Geometry: final body of the model. Coordinates: model frame, mm. A direction names the side the tool comes from. Give positions to 0.01 mm unless a question says otherwise; leave off trailing zeros. Write each loop counter-clockwise with the first axis right and the second up, starting at its lowest first coordinate (ties: lowest second). Pieces come first, ordered by that corner, then holes. Notation, with made-up numbers: M 86.5,66 L 106.5,66 A12 cw 106.5,85 Z; hole C 53,-28.5 d9. An arc over 180 degrees is marked long. Answer as a JSON object with one key per item and string values.
from build123d import *

# Parameters (mm, degrees)
F1_DEPTH  = 16
F3_DEPTH  = 8
F5_DEPTH  = 3
F7_R      = 4.4
F6_R      = 4.55
F9_ANGLE  = 90
F10_SIZE2 = 7
F10_SIZE  = 5


with BuildPart() as f1:
    # F0 (on Top) → F1 (new body)
    with BuildSketch(Plane.XY):
        with BuildLine():
            ThreePointArc((10.125, 0), (0, 10.125), (-10.125, 0))
            Line((-10.125, 0), (-10.125, -10.125))
            Line((-10.125, -10.125), (10.125, -10.125))
            Line((10.125, -10.125), (10.125, 0))
        make_face()
    extrude(amount=F1_DEPTH)

    # F2 (on face) → F3 (cut)
    with BuildSketch(Plane.XY.offset(16)):
        with BuildLine():
            ThreePointArc((7.8, 0), (0, 7.8), (-7.8, 0))
            Line((-7.8, 0), (-7.8, -10.125))
            Line((-7.8, -10.125), (7.8, -10.125))
            Line((7.8, -10.125), (7.8, 0))
        make_face()
    extrude(amount=-F3_DEPTH, mode=Mode.SUBTRACT)

    # F4 (on face) → F5 (cut)
    with BuildSketch(Plane.XY.offset(8)):
        with BuildLine():
            ThreePointArc((9.125, 0), (0, 9.125), (-9.125, 0))
            Line((-9.125, 0), (-9.125, -10.125))
            Line((-9.125, -10.125), (9.125, -10.125))
            Line((9.125, -10.125), (9.125, 0))
        make_face()
    extrude(amount=F5_DEPTH, mode=Mode.SUBTRACT)

    # F7 (on face) → F8 section 0
    with BuildSketch(Plane(origin=(0, 0, 0), x_dir=(1, 0, 0), z_dir=(0, 0, -1))):
        Circle(F7_R)
    # F6 (on face) → F8 section 1
    with BuildSketch(Plane.XY.offset(8)):
        Circle(F6_R)
    loft(mode=Mode.SUBTRACT)


with BuildPart() as f1_1:
    # F9: moved
    add(f1.part.rotate(Axis((0, -10.125, 0), (1, 0, 0)), F9_ANGLE))

    # F10
    f10_edges = [f1_1.edges().sort_by_distance(p)[0] for p in [
        (10.125, -10.125, 5.0625),
        (0, -10.125, 20.25),
        (0, -10.125, 0),
    ]]
    f10_side = f1_1.faces().sort_by_distance((0, -10.125, 19.963622))[0]
    chamfer(f10_edges, length=F10_SIZE, length2=F10_SIZE2, reference=f10_side)


solid = f1_1.part
1) Pull-direction query (Y, two-part tool) for faces 1 (the flat face through (7.66, -13.674, 6.117)), 2 (the conical face through (-0.583, -14.181, 5.687)), 3 (the flat face through (-4, -21.125, 17)); classes: pulls with the +Y half, pulls with the -Y half, needs draft (parallel to the pull), parting line crosses it, or undercut.
Geometry check:
{"face 1": "pulls with the +Y half", "face 2": "pulls with the -Y half", "face 3": "undercut"}
2) Cut plane A-A on y = -21.75. Return loops of the section in (x, z) (3 decimals).
Geometry check:
{"outline": "M -10.125,0 L -7.8,0 L -7.8,10.125 A7.8 cw 7.8,10.125 L 7.8,0 L 10.125,0 L 10.125,10.125 A10.125 ccw -10.125,10.125 Z"}
3) Cut plane B-B on z = 4.25. Return loops of the section in (x, y) (3 decimals).
Geometry check:
{"outline": "M -10.125,-26.125 L -7.8,-26.125 L -7.8,-21.125 L -9.125,-21.125 L -9.125,-18.125 L 9.125,-18.125 L 9.125,-21.125 L 7.8,-21.125 L 7.8,-26.125 L 10.125,-26.125 L 10.125,-17.125 L 5.875,-11.175 L -5.875,-11.175 L -10.125,-17.125 Z"}
4) Set-up query: faces 4 (the cylindrical face through (0.201, -19.604, 19.248)), 5 (the flat face through (-0.8, -17.9, 0)), 6 (the flat face through (7.8, -24, 5)). Return all of +Z, -Z, +X, -X, +Y, -Y with unobstructed straight access to the full face (end or side cutting, diameter ignored); none if empty.
Geometry check:
{"face 4": "-Z", "face 5": "-Z, +X, -X, +Y, -Y", "face 6": "-Z, -Y"}
5) Contact query for flat-ended pins moving along their axis: P1, Ø2, axis at x = 1.5, z = 17.5, coming from the -Y side (3 decimals); P2, Ø4, axis at x = 3.5, y = -13.5, coming from the -Z side; P3, Ø8, axis at y = -13, z = 7, coming from the +X side; P4, Ø9, axis at x = 0.5, z = 8, coming from the -Y side (3 decimals). Output: stop coordinate, or through.
Geometry check:
{"P1": "stops at y = -26.125", "P2": "stops at z = 1.16", "P3": "stops at x = 10.04", "P4": "stops at y = -18.125"}
6) Cut plane C-C on y = -19.5. Return loops of the section in (x, z) (3 decimals), and give its area (3 significant figures).
Geometry check:
{"outline": "M -10.125,0 L -9.125,0 L -9.125,10.125 A9.125 cw 9.125,10.125 L 9.125,0 L 10.125,0 L 10.125,10.125 A10.125 ccw -10.125,10.125 Z", "area": "50.5 mm2"}
7) Line query: line 1 (X direction, y = -20, z = 7.5) (3 decimals); line 2 (X direction, y = -23, z = 9) (3 decimals); line 3 (Z direction, x = -1, y = -12.5). Output: solid intervals per line, ascending. Write a range as from..to.
Geometry check:
{"line 1": "x = -10.125..-9.125, 9.125..10.125", "line 2": "x = -10.125..-7.8, 7.8..10.125", "line 3": "z = 3.3..5.79, 14.46..16.87"}
